Work out the finished part from the listing and answer in its coordinate system (mm). Face numbers are marked on the shaded views. Coordinates: 2 decimals unless noted, no trailing zeros.
```python
from build123d import *

# Parameters (mm, degrees)
F4_T     = -2.5
F5_R     = 20
F6_DEPTH = 2.5


with BuildPart() as f3:
    # F2 (on offset) → F3 section 0
    with BuildSketch(Plane.XZ.offset(250)):
        with BuildLine():
            ThreePointArc((80, 40), (68.284271, 68.284271), (40, 80))
            Line((40, 80), (-40, 80))
            ThreePointArc((-40, 80), (-68.284271, 68.284271), (-80, 40))
            Line((-80, 40), (-80, -40))
            ThreePointArc((-80, -40), (-68.284271, -68.284271), (-40, -80))
            Line((-40, -80), (40, -80))
            ThreePointArc((40, -80), (68.284271, -68.284271), (80, -40))
            Line((80, -40), (80, 40))
        make_face()
    # F0 (on Front) → F3 section 1
    with BuildSketch(Plane.XZ):
        with BuildLine():
            ThreePointArc((40, 20), (34.142136, 34.142136), (20, 40))
            Line((20, 40), (-20, 40))
            ThreePointArc((-20, 40), (-34.142136, 34.142136), (-40, 20))
            Line((-40, 20), (-40, -20))
            ThreePointArc((-40, -20), (-34.142136, -34.142136), (-20, -40))
            Line((-20, -40), (20, -40))
            ThreePointArc((20, -40), (34.142136, -34.142136), (40, -20))
            Line((40, -20), (40, 20))
        make_face()
    loft()

    # F4
    f4_openings = [f3.faces().sort_by_distance(p)[0] for p in [
        (0, -250, 0),
    ]]
    offset(amount=F4_T, openings=f4_openings)

    # F5 (on face) → F6 (cut, through all)
    with BuildSketch(Plane(origin=(0, 0, 0), x_dir=(-1, 0, 0), z_dir=(0, 1, 0))):
        Circle(F5_R)
    extrude(amount=-F6_DEPTH, mode=Mode.SUBTRACT)


solid = f3.part
```
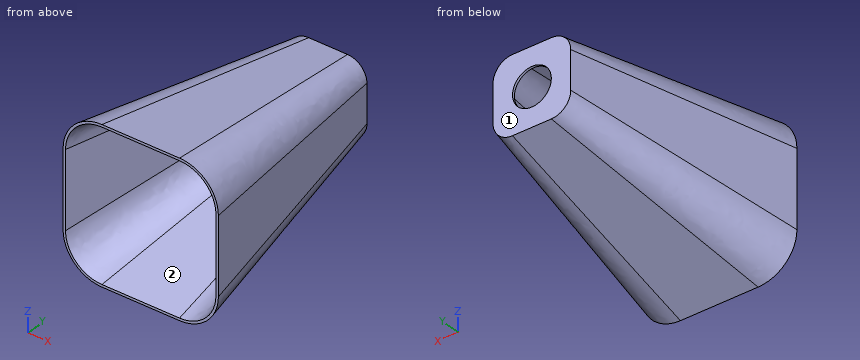
1. Determine the mould class of the marked faces 1 and 2 for opening direction Z: released by +Z, released by -Z, zero draft, split by the parting line, or undercut.
2. Straight lines are drawn through the part: probe 1 along Z at (x, y) = (-19, -234); probe 2 along Z at (x, y) = (0, -1.2); probe 3 along X at (y, z) = (-198, 58). For each, find the intervals that lie inside material, in ascending order.
3. Each of these flat-tipped pins is pushed along its axis until it touches: P1, Ø5, axis at y = -178.5, z = -2, coming from the +X side; P2, Ø3, axis at y = -71, z = -23, coming from the -X side; P3, Ø5, axis at y = -159.5, z = -52.5, coming from the -X side; P4, Ø22.5, axis at x = -0.5, z = -7.5, coming from the -Y side. Where does it stop, or does it pass through?
Answers below:
1. face 1: zero draft
1. face 2: undercut
2. probe 1: z = -77.44 to -74.91, 74.91 to 77.44
2. probe 2: z = -40.19 to -20, 20 to 40.19
2. probe 3: x = -64.01 to -60.69, 60.69 to 64.01
3. P1: stops at x = 68.96
3. P2: stops at x = -51.6
3. P3: stops at x = -60.71
3. P4: passes through
